Part model, mm, in its own coordinate system. A direction names the side the tool comes from. Give positions to 0.01 mm unless a question says otherwise; leave off trailing zeros. Write each loop counter-clockwise with the first axis right and the second up, starting at its lowest first coordinate (ties: lowest second). Pieces come first, ordered by that corner, then holes.
Autodesk Inventor part; units mm, degrees
ref_plane "YZ Plane" through (0, 0, 0) normal (1, 0, 0) x (0, 1, 0)
ref_plane "XZ Plane" through (0, 0, 0) normal (0, 1, 0) x (-1, 0, 0)
ref_plane "XY Plane" through (0, 0, 0) normal (0, 0, 1) x (1, 0, 0)
sketch "Sketch1" plane through (0, 0, 0) normal (0, 1, 0) x (-1, 0, 0)
  line L0 (-1.7321, 3) -> (1.7321, 3)
  line L1 (1.7321, 3) -> (3.4641, 0)
  line L2 (3.4641, 0) -> (1.7321, -3)
  line L3 (1.7321, -3) -> (-1.7321, -3)
  line L4 (-1.7321, -3) -> (-3.4641, 0)
  line L5 (-3.4641, 0) -> (-1.7321, 3)
  point P0 (0, 0)
  point P1 (0, 0)
  dimension "d0" = 6
extrude "Extrusion1" add sketch "Sketch1" along normal blind 30
sketch "Sketch2" plane through (0, 30, 0) normal (0, 1, 0) x (1, 0, 0)
  point P0 (0, 0)
hole "Hole1" at (0, 30, 0) direction (0, -1, 0) diameter 3.4 depth 4 tip angle 118
sketch "Sketch3" plane through (0, 0, 0) normal (0, -1, 0) x (1, 0, 0)
  point P0 (0, 0)
hole "Hole2" at (0, 0, 0) direction (0, 1, 0) diameter 3.4 depth 4 tip angle 118
properties part number "tavtarto_30mm"
1) 3-axis set-ups, long thin cutter, end or side, ignore diameter. For faces 4 (the face through (-2.6, 14.8, 1.5)), 5 (the face through (1.66, 2.03, 0.37)), 6 (the face through (1.66, 27.97, -0.37)): which of +Z, -Z, +X, -X, +Y, -Y reach the whole face in a straight line?
Answers follow:
face 4: +Z, -X, +Y, -Y
face 5: -Y
face 6: +Y
2) Saw through at B-B, the plane x = -2.5. Write the cut outline in (y, z), then the cut area to 3 significant figures.
Answers follow:
outline: (0, -1.67) - (30, -1.67) - (30, 1.67) - (0, 1.67) - close
area: 100 mm2
3) Wall check: L1, parallel to Z at x = 0, y = 2.95; L2, parallel to Y at x = 0.5, z = -0.7; L3, parallel to X at y = 4.25, z = -2.45. Give the ranges that are in metal, low to high.
Answers follow:
L1: z = -3 to -1.7, 1.7 to 3
L2: y = 4.5 to 25.5
L3: x = -2.05 to 2.05
4) Two-plate mould, pull along Z, no slides. Class faces 1 (the face through (2, 0, 1)), 2 (the face through (2.6, 14.8, 1.5)), 3 (the face through (-0.288, 25.156, -0.064)): +Z half, -Z half, draft (parallel to the pull), parting line (faces both ways), or undercut.
Answers follow:
face 1: draft
face 2: +Z half
face 3: undercut
5) Pin check, flat tips, straight feed: pin 1 Ø2 at (y, z) = (17, -1.5) entering from -X; pin 2 Ø2 at (x, z) = (0, 0) entering from -Y. Stop position of each tip, or through.
Answers follow:
pin 1: stops at x = -3.18
pin 2: stops at y = 4.42
6) Saw through at C-C, the plane z = -2.45. Write the cut outline in (x, y), then the cut area to 3 significant figures.
Answers follow:
outline: (-2.05, 0) - (2.05, 0) - (2.05, 30) - (-2.05, 30) - close
area: 123 mm2
7) Saw through at A-A, the plane y = 24.5. Write the cut outline in (x, z), then the cut area to 3 significant figures.
Answers follow:
outline: (-3.46, 0) - (-1.73, -3) - (1.73, -3) - (3.46, 0) - (1.73, 3) - (-1.73, 3) - close
area: 31.2 mm2
